Part model, mm, in its own coordinate system. Round coordinates to 2 decimals unless told otherwise and drop trailing zeros. Loops run counter-clockwise (first coordinate to the right, second up) from the corner with the lowest first, then second, coordinate; pieces in that order, holes last. Notation, with made-up numbers: M 88,-33.5 L 118,-33.5 A21 ccw 118,-28.5 Z; hole C -15,-24 d9. An arc over 180 degrees is marked long. Answer as CSV lines item,"result". Start each with the question number.
Item 1: Band-saw the part on A-A (x = -40). Give the cut face in (y, z), and give its area (3 significant figures).
Item 2: Band-saw the part on C-C (z = -5). Give the cut face in (x, y).
Item 3: Wall check: line 1 (Z direction, x = -5, y = 4.5); line 2 (X direction, y = 4.85, z = 71.5); line 3 (X direction, y = 5.4, z = -37). Give the ranges that are in metal, low to high.
Item 4: Band-saw the part on B-B (y = 4.85). Count the separate pieces of the cut face and the enclosed holes in it, and give its area (3 significant figures).
Item 5: Drop flat-ended pins along their axis: pin 1 Ø4.5 at (x, z) = (65.86, 110.78) entering from -Y; pin 2 Ø2 at (x, y) = (34.5, 4.5) entering from -Z; pin 3 Ø3 at (x, y) = (81, 3) entering from +Z; pin 4 Ø2 at (x, y) = (-22, 5.5) entering from +Z. Give the stop position or say it passes through.
```python
from build123d import *

# Parameters (mm, degrees)
SKETCH1_R           = 2.5
SKETCH1_R_2         = 2
SKETCH1_W           = 20
SKETCH1_H           = 6
SKETCH1_W_2         = 10
SKETCH1_W_3         = 6
SKETCH1_H_2         = 15.5
SKETCH1_H_3         = 10
BOSS_EXTRUDE1_DEPTH = 6


with BuildPart() as part:
    # Sketch1 → Boss-Extrude1 (new body)
    with BuildSketch(Plane(origin=(0, 0, 0), x_dir=(1, 0, 0), z_dir=(0, 1, 0))):
        with BuildLine():
            Line((-45, 125.078427477), (-45, 120.078427477))
            Line((-45, 120.078427477), (45, 120.078427477))
            Line((45, 120.078427477), (45, 125.078427477))
            ThreePointArc((45, 125.078427477), (73.284271247, 113.362698724), (85, 85.078427477))
            Line((85, 85.078427477), (75, 85.078427477))
            Line((75, 85.078427477), (75, -89.921572523))
            Line((75, -89.921572523), (85, -89.921572523))
            Line((85, -89.921572523), (85, -116.261318485))
            Line((85, -116.261318485), (70.323194947, -124.644732005))
            Line((70.323194947, -124.644732005), (55.323194947, -124.450192088))
            Line((55.323194947, -124.450192088), (51.474604803, -120.914658182))
            Line((51.474604803, -120.914658182), (28.549864753, -120.914658182))
            Line((28.549864753, -120.914658182), (25.014330847, -124.450192088))
            Line((25.014330847, -124.450192088), (-24.985669153, -124.450192088))
            Line((-24.985669153, -124.450192088), (-28.521203059, -120.914658182))
            Line((-28.521203059, -120.914658182), (-51.44594311, -120.914658182))
            Line((-51.44594311, -120.914658182), (-54.981477016, -124.450192088))
            Line((-54.981477016, -124.450192088), (-69.981477016, -124.450192088))
            Line((-69.981477016, -124.450192088), (-85, -116.261318485))
            Line((-85, -116.261318485), (-85, -89.921572523))
            Line((-85, -89.921572523), (-75, -89.921572523))
            Line((-75, -89.921572523), (-75, 85.078427477))
            Line((-75, 85.078427477), (-85, 85.078427477))
            ThreePointArc((-85, 85.078427477), (-73.284271247, 113.362698724), (-45, 125.078427477))
        make_face()
        with Locations(Location((-45, 85.078427477, 0), (0, 0, 270))):
            Circle(SKETCH1_R, mode=Mode.SUBTRACT)
        with Locations(Location((45, 85.078427477, 0), (0, 0, 270))):
            Circle(SKETCH1_R, mode=Mode.SUBTRACT)
        with Locations(Location((-65.857864376, -110.779436899, 0), (0, 0, 270))):
            Circle(SKETCH1_R, mode=Mode.SUBTRACT)
        with Locations(Location((65.857864376, -110.779436899, 0), (0, 0, 90))):
            Circle(SKETCH1_R, mode=Mode.SUBTRACT)
        with Locations(Location((19.5, 65.078427477, 0), (0, 0, 270))):
            Circle(SKETCH1_R_2, mode=Mode.SUBTRACT)
        with Locations(Location((-19.5, 65.078427477, 0), (0, 0, 270))):
            Circle(SKETCH1_R_2, mode=Mode.SUBTRACT)
        Polygon((50.571600169, 109.810660524), (54.814240856, 114.053301211), (68.95637648, 99.911165587), (64.713735792, 95.6685249), align=None, mode=Mode.SUBTRACT)
        with Locations((0, 113.078427477)):
            Rectangle(SKETCH1_W, SKETCH1_H, mode=Mode.SUBTRACT)
        Polygon((-50.11039508, 110.271865613), (-64.252530704, 96.129729989), (-68.495171391, 100.372370676), (-54.353035767, 114.5145063), align=None, mode=Mode.SUBTRACT)
        with Locations((-39.983573085, -110.414658182)):
            Rectangle(SKETCH1_W_2, SKETCH1_H, mode=Mode.SUBTRACT)
        with Locations((40.012234778, -110.414658182)):
            Rectangle(SKETCH1_W_2, SKETCH1_H, mode=Mode.SUBTRACT)
        with Locations((54, -74.171572523)):
            Rectangle(SKETCH1_W_3, SKETCH1_H_2, mode=Mode.SUBTRACT)
        with Locations((-54, -74.171572523)):
            Rectangle(SKETCH1_W_3, SKETCH1_H_2, mode=Mode.SUBTRACT)
        with Locations((54, 78.578427477)):
            Rectangle(SKETCH1_W_3, SKETCH1_H_3, mode=Mode.SUBTRACT)
        with Locations((-54, 78.578427477)):
            Rectangle(SKETCH1_W_3, SKETCH1_H_3, mode=Mode.SUBTRACT)
    extrude(amount=BOSS_EXTRUDE1_DEPTH)


solid = part.part
```
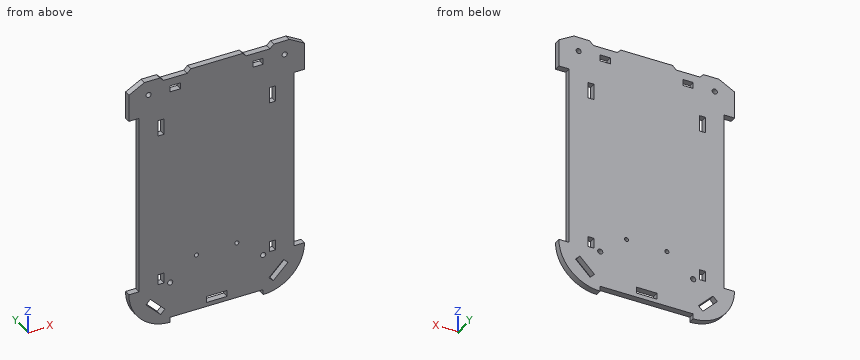
Answer block:
1,outline,"M 0,-120.08 L 6,-120.08 L 6,107.41 L 0,107.41 Z; M 0,113.41 L 6,113.41 L 6,120.91 L 0,120.91 Z"
1,area,"1,410 mm^2"
2,outline,"M -75,0 L 75,0 L 75,6 L -75,6 Z"
3,line 1,"z = -120.08 to -116.08, -110.08 to 124.45"
3,line 2,"x = -75 to -57, -51 to 51, 57 to 75"
3,line 3,"x = -75 to 75"
4,separate pieces,"1"
4,enclosed holes,"15"
4,area,"36,600 mm^2"
5,pin 1,"passes through"
5,pin 2,"stops at z = -120.08"
5,pin 3,"stops at z = 119.4"
5,pin 4,"stops at z = 124.45"
